```python
from build123d import *

# Parameters (mm, degrees)
SKETCH1_W           = 76.2
SKETCH1_H           = 31.75
BOSS_EXTRUDE1_DEPTH = 25.4
M12_TAPPED_HOLE2_D  = 10.2
M12_TAPPED_HOLE1_D  = 10.2


with BuildPart() as part:
    # Sketch1 → Boss-Extrude1 (new body)
    with BuildSketch(Plane.XY):
        with Locations((38.1, 15.875)):
            Rectangle(SKETCH1_W, SKETCH1_H)
    extrude(amount=BOSS_EXTRUDE1_DEPTH)

    # M12 Tapped Hole2 (through all)
    with Locations(Plane.XY.offset(25.4)):
        with Locations((13.1, 15.875), (63.1, 15.875)):
            Hole(M12_TAPPED_HOLE2_D / 2)

    # M12 Tapped Hole1 (through all)
    with Locations(Plane(origin=(0, 31.75, 0), x_dir=(1, 0, 0), z_dir=(0, 1, 0))):
        with Locations((38.1, -12.7)):
            Hole(M12_TAPPED_HOLE1_D / 2)


solid = part.part
```
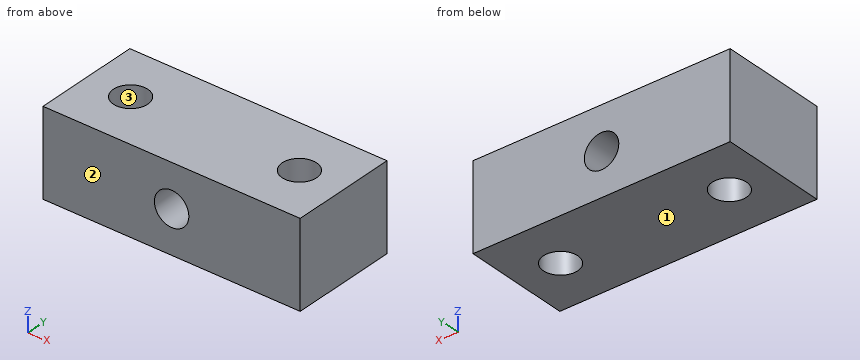
Work out the finished part from the listing and answer in its coordinate system (mm). Face numbers are marked on the shaded views. Round coordinates to 2 decimals unless told otherwise and drop trailing zeros. Write each loop counter-clockwise with the first axis right and the second up, starting at its lowest first coordinate (ties: lowest second). Pieces come first, ordered by that corner, then holes.
1) A cutting plane is placed at A-A on z = 12.7. Determine the outline of the cut face in (x, y) (3 decimals).
2) Determine the mould class of the marked faces 1, 2 and 3 for opening direction Y: pulls with the +Y half, pulls with the -Y half, needs draft (parallel to the pull), parting line crosses it, or undercut.
3) A cutting plane is placed at C-C on y = 14. Determine the outline of the cut face in (x, z).
4) A cutting plane is placed at D-D on x = 63.1. Determine the outline of the cut face in (y, z) (3 decimals).
5) A cutting plane is placed at B-B on x = 38.1. Determine the outline of the cut face in (y, z), and give its area (3 significant figures).
6) Consider probe 1 along Y at (x, z) = (63.1, 11.5) (3 decimals); probe 2 along Z at (x, y) = (38.1, 16.5); probe 3 along X at (y, z) = (13, 21.25). Determine where each line is inside the solid, lowest interval first.
Entries:
1. outline: (0, 0) - (33, 0) - (33, 31.75) - (0, 31.75) - close; (43.2, 0) - (76.2, 0) - (76.2, 31.75) - (43.2, 31.75) - close; hole circle Ø10.2 at (13.1, 15.875); hole circle Ø10.2 at (63.1, 15.875)
2. face 1: needs draft
2. face 2: pulls with the -Y half
2. face 3: undercut
3. outline: (0, 0) - (8.36, 0) - (8.36, 25.4) - (0, 25.4) - close; (17.84, 0) - (58.36, 0) - (58.36, 25.4) - (17.84, 25.4) - close; (67.84, 0) - (76.2, 0) - (76.2, 25.4) - (67.84, 25.4) - close; hole circle Ø10.2 at (38.1, 12.7)
4. outline: (0, 0) - (10.775, 0) - (10.775, 25.4) - (0, 25.4) - close; (20.975, 0) - (31.75, 0) - (31.75, 25.4) - (20.975, 25.4) - close
5. outline: (0, 0) - (31.75, 0) - (31.75, 7.6) - (0, 7.6) - close; (0, 17.8) - (31.75, 17.8) - (31.75, 25.4) - (0, 25.4) - close
5. area: 483 mm2
6. probe 1: y = 0 to 10.775, 20.975 to 31.75
6. probe 2: z = 0 to 7.6, 17.8 to 25.4
6. probe 3: x = 0 to 8.89, 17.31 to 58.89, 67.31 to 76.2
